Job drawing, mm, ordinate dimensions from the low corner. One solid piece. A direction names the side the tool comes from. Give positions to 0.01 mm unless a question says otherwise; leave off trailing zeros. Write each loop counter-clockwise with the first axis right and the second up, starting at its lowest first coordinate (ties: lowest second). Pieces come first, ordered by that corner, then holes. Notation, with made-up numbers: (-40, 87) -> (-30, 87) arc R29 ccw to (-30, 122) -> close; hole circle Ø2 at (87, -5). An arc over 180 degrees is marked (long way). One line per question, with ' | ' between items. Start each with the question number.
(1) Tool access for the marked faces 4 and 5: list every direction of +Z, -Z, +X, -X, +Y, -Y with a clear straight run to the whole face (end or side of a thin tool).
(2) Pull direction X, two halves, no side cores. Call the marked faces 1, 2 and 3: released by +X, released by -X, zero draft, split by the parting line, or undercut.
(3) Band-saw the part on A-A, the plane y = 12. Give the cut face in (x, z), and give its area (3 significant figures).
(4) Drill centre lines: probe 1 along X at (y, z) = (22, 44.5); probe 2 along X at (y, z) = (41.5, 52.5) (1 decimal); probe 3 along Y at (x, z) = (36, 21). Where is each one in solid material? Low to high. Write a range as from..to.
(5) Band-saw the part on B-B, the plane z = 7.5. Count the separate pieces of the cut face and the enclosed holes in it, and give its area (3 significant figures).
(6) Band-saw the part on D-D, the plane z = 38. Give the cut face in (x, y), and give its area (3 significant figures).
(7) Pin check, flat tips, straight feed: P1, Ø1.5, axis at x = 23, z = 55.5, coming from the -Y side; P2, Ø2.5, axis at x = 100.965, z = 65.715, coming from the -Y side; P3, Ø6.5, axis at x = 99.5, z = 64.5, coming from the +Y side (1 decimal); P4, Ø3, axis at x = 6, y = 6, coming from the -Z side (1 decimal). Stop position of each tip, or through.
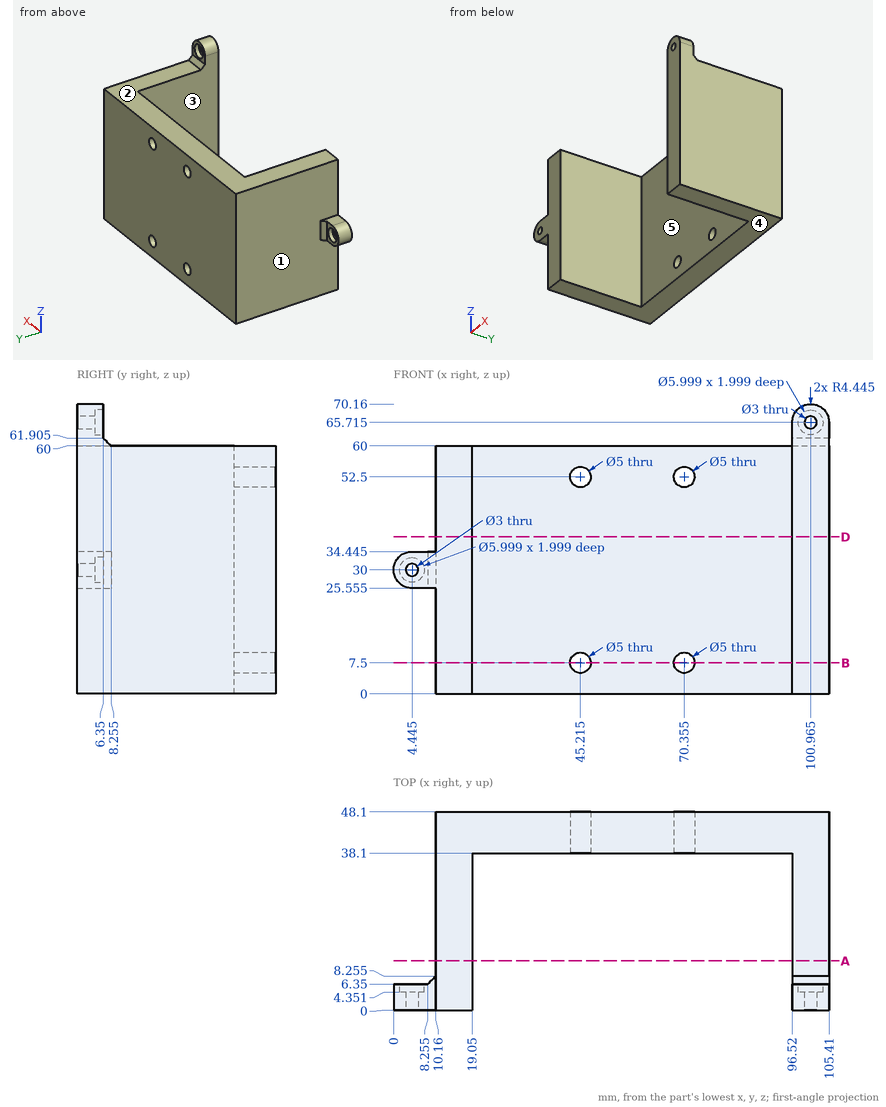
Results:
1) face 4: -Z, +X, -X, +Y, -Y | face 5: +Z, -Z, -Y
2) face 1: released by -X | face 2: zero draft | face 3: undercut
3) outline: (10.16, 0) -> (19.05, 0) -> (19.05, 60) -> (10.16, 60) -> close; (96.52, 0) -> (105.41, 0) -> (105.41, 60) -> (96.52, 60) -> close | area: 1,070 mm²
4) probe 1: x = 10.16..19.05, 96.52..105.41 | probe 2: x = 10.2..42.7, 47.7..67.9, 72.9..105.4 | probe 3: y = 38.1..48.1
5) separate pieces: 3 | enclosed holes: 0 | area: 1,530 mm²
6) outline: (10.16, 0) -> (19.05, 0) -> (19.05, 38.1) -> (96.52, 38.1) -> (96.52, 0) -> (105.41, 0) -> (105.41, 48.1) -> (10.16, 48.1) -> close | area: 1,630 mm²
7) P1: stops at y = 38.1 | P2: passes through | P3: stops at y = 7 | P4: stops at z = 25.6
